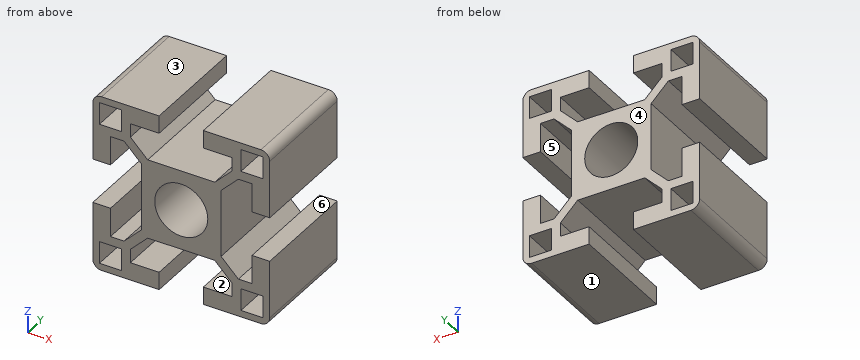
```python
from build123d import *

# Parameters (mm, degrees)
F0_W     = 5
F0_H     = 5
F0_R     = 6
F1_DEPTH = 25


with BuildPart() as f1:
    # F0 (on Front) → F1 (new body)
    with BuildSketch(Plane.XZ):
        with BuildLine():
            Line((5, -20), (18, -20))
            ThreePointArc((18, -20), (19.414214, -19.414214), (20, -18))
            Line((20, -18), (20, -5))
            Line((20, -5), (16, -5))
            Line((16, -5), (16, -11.5))
            Line((16, -11.5), (12.914214, -11.5))
            Line((12.914214, -11.5), (9, -7.585786))
            Line((9, -7.585786), (9, 0))
            Line((9, 0), (9, 7.585786))
            Line((9, 7.585786), (12.914214, 11.5))
            Line((12.914214, 11.5), (16, 11.5))
            Line((16, 11.5), (16, 5))
            Line((16, 5), (20, 5))
            Line((20, 5), (20, 18))
            ThreePointArc((20, 18), (19.414214, 19.414214), (18, 20))
            Line((18, 20), (5, 20))
            Line((5, 20), (5, 16))
            Line((5, 16), (11.5, 16))
            Line((11.5, 16), (11.5, 12.914214))
            Line((11.5, 12.914214), (7.585786, 9))
            Line((7.585786, 9), (0, 9))
            Line((0, 9), (-7.585786, 9))
            Line((-7.585786, 9), (-11.5, 12.914214))
            Line((-11.5, 12.914214), (-11.5, 16))
            Line((-11.5, 16), (-5, 16))
            Line((-5, 16), (-5, 20))
            Line((-5, 20), (-18, 20))
            ThreePointArc((-18, 20), (-19.414214, 19.414214), (-20, 18))
            Line((-20, 18), (-20, 5))
            Line((-20, 5), (-16, 5))
            Line((-16, 5), (-16, 11.5))
            Line((-16, 11.5), (-12.914214, 11.5))
            Line((-12.914214, 11.5), (-9, 7.585786))
            Line((-9, 7.585786), (-9, 0))
            Line((-9, 0), (-9, -7.585786))
            Line((-9, -7.585786), (-12.914214, -11.5))
            Line((-12.914214, -11.5), (-16, -11.5))
            Line((-16, -11.5), (-16, -5))
            Line((-16, -5), (-20, -5))
            Line((-20, -5), (-20, -18))
            ThreePointArc((-20, -18), (-19.414214, -19.414214), (-18, -20))
            Line((-18, -20), (-5, -20))
            Line((-5, -20), (-5, -16))
            Line((-5, -16), (-11.5, -16))
            Line((-11.5, -16), (-11.5, -12.914214))
            Line((-11.5, -12.914214), (-7.585786, -9))
            Line((-7.585786, -9), (0, -9))
            Line((0, -9), (7.585786, -9))
            Line((7.585786, -9), (11.5, -12.914214))
            Line((11.5, -12.914214), (11.5, -16))
            Line((11.5, -16), (5, -16))
            Line((5, -16), (5, -20))
        make_face()
        with Locations((-16, -16)):
            Rectangle(F0_W, F0_H, mode=Mode.SUBTRACT)
        with Locations((16, -16)):
            Rectangle(F0_W, F0_H, mode=Mode.SUBTRACT)
        with Locations((-16, 16)):
            Rectangle(F0_W, F0_H, mode=Mode.SUBTRACT)
        Circle(F0_R, mode=Mode.SUBTRACT)
        with Locations((16, 16)):
            Rectangle(F0_W, F0_H, mode=Mode.SUBTRACT)
    extrude(amount=F1_DEPTH)


solid = f1.part
```
For this review, take the finished solid that the model builds, in its own axes (mm). Face numbers are marked on the shaded views. A direction names the side the tool comes from. Round coordinates to 2 decimals unless told otherwise and drop trailing zeros. Write each loop counter-clockwise with the first axis right and the second up, starting at its lowest first coordinate (ties: lowest second). Pieces come first, ordered by that corner, then holes. Notation, with made-up numbers: (9, 85) - (34, 85) arc R28 cw to (34, 110) - close; hole circle Ø4 at (70, 3). An arc over 180 degrees is marked (long way). Answer as a JSON object with one key per item and string values.
1. Draft analysis for pull direction Z (two halves, no side actions). For the marked faces 1, 2 and 3, state which applies: +Z half, -Z half, draft (parallel to the pull), parting line (faces both ways), or undercut.
Response values:
{"face 1": "-Z half", "face 2": "undercut", "face 3": "+Z half"}
2. We need section B-B on x = 0. Give the boundary of the cut face in (y, z).
Response values:
{"outline": "(-25, -9) - (0, -9) - (0, -6) - (-25, -6) - close; (-25, 6) - (0, 6) - (0, 9) - (-25, 9) - close"}
3. We need section D-D on z = 9.5. Give the boundary of the cut face in (x, y).
Response values:
{"outline": "(-20, -25) - (-16, -25) - (-16, 0) - (-20, 0) - close; (-10.91, -25) - (-8.09, -25) - (-8.09, 0) - (-10.91, 0) - close; (8.09, -25) - (10.91, -25) - (10.91, 0) - (8.09, 0) - close; (16, -25) - (20, -25) - (20, 0) - (16, 0) - close"}
4. For pin 1 Ø7.5 at (y, z) = (-17, 0) entering from -X, flat-tipped, find the tip position at first contact; note if it passes through.
Response values:
{"pin 1": "stops at x = -9"}
5. To check wall thickness, follow line 1 along Z through (x, y) = (-18, -13.75); line 2 along Z through (x, y) = (-7.5, -14). State the ranges of each line that lie inside material, in increasing order.
Response values:
{"line 1": "z = -20 to -18.5, -13.5 to -5, 5 to 13.5, 18.5 to 20", "line 2": "z = -20 to -16, -9 to 9, 16 to 20"}
6. We need section C-C on x = -6.5. Give the boundary of the cut face in (y, z).
Response values:
{"outline": "(-25, -20) - (0, -20) - (0, -16) - (-25, -16) - close; (-25, -9) - (0, -9) - (0, 9) - (-25, 9) - close; (-25, 16) - (0, 16) - (0, 20) - (-25, 20) - close"}
7. Tool access review of the marked faces 4, 5 and 6: name each direction out of +Z, -Z, +X, -X, +Y, -Y from which nothing blocks a thin tool from reaching the whole face with its end or side.
Response values:
{"face 4": "+Z, -Z, +X, -X, +Y", "face 5": "+Y, -Y", "face 6": "+X, +Y, -Y"}
8. We need section A-A on z = 0. Give the boundary of the cut face in (x, y), then the cut area to 3 significant figures.
Response values:
{"outline": "(-9, -25) - (-6, -25) - (-6, 0) - (-9, 0) - close; (6, -25) - (9, -25) - (9, 0) - (6, 0) - close", "area": "150 mm2"}
